```python
from build123d import *

# Parameters (mm, degrees)
PAD_DEPTH       = 140
SKETCH001_W     = 3
SKETCH001_H     = 5
PAD001_DEPTH    = 58
SKETCH002_W     = 2
SKETCH002_H     = 3
POCKET_DEPTH    = 58
SKETCH003_W     = 3
SKETCH003_H     = 5
PAD002_DEPTH    = 58
SKETCH004_W     = 2
SKETCH004_H     = 3
POCKET001_DEPTH = 58
PAD003_DEPTH    = 32
PAD004_DEPTH    = 32
PAD005_DEPTH    = 17
PAD006_DEPTH    = 17
PAD007_DEPTH    = 53
POCKET002_DEPTH = 134
POCKET003_DEPTH = 57
POCKET004_DEPTH = 32
POCKET005_DEPTH = 17
POCKET006_DEPTH = 17
POCKET007_DEPTH = 32


with BuildPart() as part:
    # Sketch → Pad (new body)
    with BuildSketch(Plane.XY):
        Polygon((0, 0), (15, 0), (15, -2), (14, -3), (1, -3), (0, -2), align=None)
    extrude(amount=PAD_DEPTH)

    # Sketch001 (on Face2 of Pad) → Pad001 (join)
    with BuildSketch(Plane.YZ):
        with Locations((-1.5, 137.5)):
            Rectangle(SKETCH001_W, SKETCH001_H)
    extrude(amount=PAD001_DEPTH)

    # Sketch002 (on Face15 of Pad001) → Pocket (cut)
    with BuildSketch(Plane.YZ.offset(58)):
        with Locations((-1, 138.5)):
            Rectangle(SKETCH002_W, SKETCH002_H)
    extrude(amount=-POCKET_DEPTH, mode=Mode.SUBTRACT)

    # Sketch003 (on Face3 of Pocket) → Pad002 (join)
    with BuildSketch(Plane.YZ):
        with Locations((-1.5, 2.5)):
            Rectangle(SKETCH003_W, SKETCH003_H)
    extrude(amount=PAD002_DEPTH)

    # Sketch004 (on Face9 of Pad002) → Pocket001 (cut)
    with BuildSketch(Plane.YZ.offset(58)):
        with Locations((-1, 1.5)):
            Rectangle(SKETCH004_W, SKETCH004_H)
    extrude(amount=-POCKET001_DEPTH, mode=Mode.SUBTRACT)

    # Sketch005 (on Face9 of Pocket001) → Pad003 (join)
    with BuildSketch(Plane.YZ):
        Polygon((0, 31), (-2, 31), (-3, 32), (-3, 45), (-2, 46), (0, 46), align=None)
    extrude(amount=PAD003_DEPTH)

    # Sketch006 (on Face30 of Pad003) → Pad004 (join)
    with BuildSketch(Plane.YZ):
        Polygon((0, 116), (0, 101), (-2, 101), (-3, 102), (-3, 115), (-2, 116), align=None)
    extrude(amount=PAD004_DEPTH)

    # Sketch007 (on Face28 of Pad004) → Pad005 (join)
    with BuildSketch(Plane.YZ.offset(32)):
        Polygon((0, 48), (0, 33), (-2, 33), (-3, 34), (-3, 47), (-2, 48), align=None)
    extrude(amount=PAD005_DEPTH)

    # Sketch008 (on Face56 of Pad005) → Pad006 (join)
    with BuildSketch(Plane.YZ.offset(32)):
        Polygon((-2, 114), (0, 114), (0, 99), (-2, 99), (-3, 100), (-3, 113), align=None)
    extrude(amount=PAD006_DEPTH)

    # Sketch009 (on Face40 of Pad006) → Pad007 (join)
    with BuildSketch(Plane.XY.offset(47)):
        Polygon((43, 0), (58, 0), (58, -2), (57, -3), (44, -3), (43, -2), align=None)
    extrude(amount=PAD007_DEPTH)

    # Sketch010 (on Face87 of Pad007) → Pocket002 (cut)
    with BuildSketch(Plane.XY.offset(137)):
        Polygon((2.5, -2), (12.5, -2), (12.5, -1.5), (12, -1.5), (12, 0), (3, 0), (3, -1.5), (2.5, -1.5), align=None)
    extrude(amount=-POCKET002_DEPTH, mode=Mode.SUBTRACT)

    # Sketch011 (on Face103 of Pocket002) → Pocket003 (cut)
    with BuildSketch(Plane.XY.offset(102)):
        Polygon((55.5, -2), (45.5, -2), (45.5, -1.5), (46, -1.5), (46, 0), (55, 0), (55, -1.5), (55.5, -1.5), align=None)
    extrude(amount=-POCKET003_DEPTH, mode=Mode.SUBTRACT)

    # Sketch012 (on Face112 of Pocket003) → Pocket004 (cut)
    with BuildSketch(Plane(origin=(0, 0, 0), x_dir=(0, -1, 0), z_dir=(-1, 0, 0))):
        Polygon((2, 113.5), (1.5, 113.5), (1.5, 113), (0, 113), (0, 104.04), (1.5, 104.04), (1.5, 103.5), (2, 103.5), align=None)
    extrude(amount=-POCKET004_DEPTH, mode=Mode.SUBTRACT)

    # Sketch013 (on Face70 of Pocket004) → Pocket005 (cut)
    with BuildSketch(Plane(origin=(32, 0, 0), x_dir=(0, -1, 0), z_dir=(-1, 0, 0))):
        Polygon((0, 111), (1.5, 111), (1.5, 111.5), (2, 111.5), (2, 101.5), (1.5, 101.5), (1.5, 102), (0, 102), align=None)
    extrude(amount=-POCKET005_DEPTH, mode=Mode.SUBTRACT)

    # Sketch014 (on Face59 of Pocket005) → Pocket006 (cut)
    with BuildSketch(Plane(origin=(32, 0, 0), x_dir=(0, -1, 0), z_dir=(-1, 0, 0))):
        Polygon((0, 45), (1.5, 45), (1.5, 45.5), (2, 45.5), (2, 35.5), (1.5, 35.5), (1.5, 36), (0, 36), align=None)
    extrude(amount=-POCKET006_DEPTH, mode=Mode.SUBTRACT)

    # Sketch015 (on Face127 of Pocket006) → Pocket007 (cut)
    with BuildSketch(Plane(origin=(0, 0, 0), x_dir=(0, -1, 0), z_dir=(-1, 0, 0))):
        Polygon((2, 33.5), (1.5, 33.5), (1.5, 34), (0, 34), (0, 43), (1.5, 43), (1.5, 43.5), (2, 43.5), align=None)
    extrude(amount=-POCKET007_DEPTH, mode=Mode.SUBTRACT)


solid = part.part
```
Design review of the part built by this model. Coordinates are the model's own, in mm. A direction names the side the tool comes from. Give positions to 0.01 mm unless a question says otherwise; leave off trailing zeros. Order: outer loops, then holes, each group sorted by start corner. A loop starts at its lowest first (then second) coordinate and runs counter-clockwise, first axis right, second up. Notation, with made-up numbers: (-5, 72.5) -> (50, 72.5) arc R33 ccw to (50, 109.5) -> close; hole circle Ø4 at (50.25, 1.5). An arc over 180 degrees is marked (long way). Write item = value, one per line. Start each with the question number.
(1) Mouldability with a two-part tool opening along Z and no side actions: class faces 1 (the face through (1, 0, 125)), 2 (the face through (49, -2.5, 38.5)) as +Z half, -Z half, draft (parallel to the pull), parting line (faces both ways), or undercut.
(2) To check wall thickness, follow line 1 along X through (y, z) = (-1, 68); line 2 along Z through (x, y) = (41, -0.4); line 3 along X through (y, z) = (-1.9, 72.5). State the ranges of each line that lie inside material, in increasing order.
(3) We need section B-B on x = 40. State how many separate pieces and enclosed holes the cut face has, plus the area to 3 significant figures.
(4) For pin 1 (0.6 mm diameter, centred on y = -2, z = 25.5, fed in from +X); pin 2 (1 mm diameter, centred on x = 16, z = 39, fed in from +Y); pin 3 (0.6 mm diameter, centred on y = -1.5, z = 85, fed in from -X); pin 4 (0.6 mm diameter, centred on y = -0.5, z = 34.5, fed in from -X), all flat-tipped, find the tip position at first contact; note any pin that passes through.
(5) We need section D-D on z = 12. Write out the cut boundary in (x, y).
(6) We need section A-A on z = 86. Write out the cut boundary in (x, y).
(7) For faces 3 (the face through (56, 0, 74)), 4 (the face through (49, -2.5, 108.7)), list the 3-axis set-ups (+Z, -Z, +X, -X, +Y, -Y) from which the entire face can be reached by the end or side of a thin tool; tool diameter is ignored.
Numbers:
q1.face_1 = draft
q1.face_2 = undercut
q2.line_1 = 0 to 3, 12 to 15, 43 to 46, 55 to 58
q2.line_2 = 3 to 5, 33 to 36, 45 to 48, 99 to 102, 111 to 114, 135 to 137
q2.line_3 = 0 to 2.5, 12.5 to 15, 43 to 45.5, 55.5 to 58
q3.separate_pieces = 4
q3.enclosed_holes = 0
q3.area = 69.0 mm^2
q4.pin_1 = 15
q4.pin_2 = -2
q4.pin_3 = 0
q4.pin_4 = 32
q5.outline = (0, -2) -> (1, -3) -> (14, -3) -> (15, -2) -> (15, 0) -> (12, 0) -> (12, -1.5) -> (12.5, -1.5) -> (12.5, -2) -> (2.5, -2) -> (2.5, -1.5) -> (3, -1.5) -> (3, 0) -> (0, 0) -> close
q6.outline = (0, -2) -> (1, -3) -> (14, -3) -> (15, -2) -> (15, 0) -> (12, 0) -> (12, -1.5) -> (12.5, -1.5) -> (12.5, -2) -> (2.5, -2) -> (2.5, -1.5) -> (3, -1.5) -> (3, 0) -> (0, 0) -> close; (43, -2) -> (44, -3) -> (57, -3) -> (58, -2) -> (58, 0) -> (55, 0) -> (55, -1.5) -> (55.5, -1.5) -> (55.5, -2) -> (45.5, -2) -> (45.5, -1.5) -> (46, -1.5) -> (46, 0) -> (43, 0) -> close
q7.face_3 = +Z, -Z, +X, -X, +Y
q7.face_4 = +X, +Y, -Y
